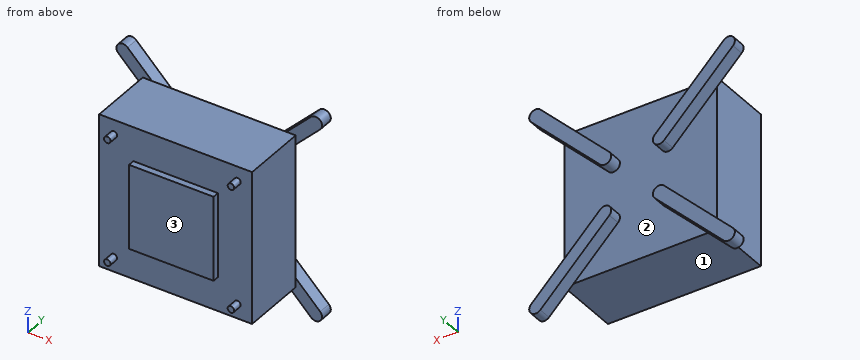
from build123d import *

# Parameters (mm, degrees)
ESQUISSE1_W        = 47
ESQUISSE1_H        = 47
BOSS_EXTRU_1_DEPTH = 20
ESQUISSE2_R        = 1
BOSS_EXTRU_2_DEPTH = 3
BOSS_EXTRU_3_DEPTH = 4
ESQUISSE4_W        = 26
ESQUISSE4_H        = 26
BOSS_EXTRU_4_DEPTH = 2


with BuildPart() as part:
    # Esquisse1 → Boss.-Extru.1 (new body)
    with BuildSketch(Plane(origin=(0, 0, 0), x_dir=(1, 0, 0), z_dir=(0, 1, 0))):
        Rectangle(ESQUISSE1_W, ESQUISSE1_H)
    extrude(amount=BOSS_EXTRU_1_DEPTH)

    # Esquisse2 → Boss.-Extru.2 (add)
    with BuildSketch(Plane.XZ):
        with Locations((19, -19)):
            Circle(ESQUISSE2_R)
        with Locations((-19, -19)):
            Circle(ESQUISSE2_R)
        with Locations((-19, 19)):
            Circle(ESQUISSE2_R)
        with Locations((19, 19)):
            Circle(ESQUISSE2_R)
    extrude(amount=BOSS_EXTRU_2_DEPTH)

    # Esquisse3 → Boss.-Extru.3 (add)
    with BuildSketch(Plane(origin=(0, 20, 0), x_dir=(1, 0, 0), z_dir=(0, 1, 0))):
        with BuildLine():
            Line((9.807611845, -6.97918472), (31.02081528, -28.192388155))
            ThreePointArc((31.02081528, -28.192388155), (31.02081528, -31.02081528), (28.192388155, -31.02081528))
            Line((28.192388155, -31.02081528), (6.97918472, -9.807611845))
            ThreePointArc((6.97918472, -9.807611845), (6.97918472, -6.97918472), (9.807611845, -6.97918472))
        make_face()
        with BuildLine():
            Line((9.807611845, 6.97918472), (31.02081528, 28.192388155))
            ThreePointArc((31.02081528, 28.192388155), (31.02081528, 31.02081528), (28.192388155, 31.02081528))
            Line((28.192388155, 31.02081528), (6.97918472, 9.807611845))
            ThreePointArc((6.97918472, 9.807611845), (6.97918472, 6.97918472), (9.807611845, 6.97918472))
        make_face()
        with BuildLine():
            Line((-9.807611845, -6.97918472), (-31.02081528, -28.192388155))
            ThreePointArc((-31.02081528, -28.192388155), (-31.02081528, -31.02081528), (-28.192388155, -31.02081528))
            Line((-28.192388155, -31.02081528), (-6.97918472, -9.807611845))
            ThreePointArc((-6.97918472, -9.807611845), (-6.97918472, -6.97918472), (-9.807611845, -6.97918472))
        make_face()
        with BuildLine():
            Line((-9.807611845, 6.97918472), (-31.02081528, 28.192388155))
            ThreePointArc((-31.02081528, 28.192388155), (-31.02081528, 31.02081528), (-28.192388155, 31.02081528))
            Line((-28.192388155, 31.02081528), (-6.97918472, 9.807611845))
            ThreePointArc((-6.97918472, 9.807611845), (-6.97918472, 6.97918472), (-9.807611845, 6.97918472))
        make_face()
    extrude(amount=BOSS_EXTRU_3_DEPTH)

    # Esquisse4 → Boss.-Extru.4 (add)
    with BuildSketch(Plane.XZ):
        Rectangle(ESQUISSE4_W, ESQUISSE4_H)
    extrude(amount=BOSS_EXTRU_4_DEPTH)


solid = part.part
Here's how the part is built. I have some questions about the finished solid (model axes, mm). Face numbers are marked on the shaded views. Round coordinates to 2 decimals unless told otherwise and drop trailing zeros. Order: outer loops, then holes, each group sorted by start corner. A loop starts at its lowest first (then second) coordinate and runs counter-clockwise, first axis right, second up. Notation, with made-up numbers: (-26.5, 72) -> (-8.5, 72) arc R30 cw to (-8.5, 97) -> close; hole circle Ø11 at (81, 28.5). An arc over 180 degrees is marked (long way). Return JSON: item names as keys, results as strings.
Q1. If we section it at C-C on z = -19: List the corners of the cut face in (x, y) for me, plus the area to 3 significant figures.
Filled sheet:
{"outline": "(-23.5, 0) -> (-20, 0) -> (-20, -3) -> (-18, -3) -> (-18, 0) -> (18, 0) -> (18, -3) -> (20, -3) -> (20, 0) -> (23.5, 0) -> (23.5, 20) -> (21.83, 20) -> (21.83, 24) -> (16.17, 24) -> (16.17, 20) -> (-16.17, 20) -> (-16.17, 24) -> (-21.83, 24) -> (-21.83, 20) -> (-23.5, 20) -> close", "area": "997 mm^2"}
Q2. If we section it at B-B on x = -2: List the corners of the cut face in (y, z) for me.
Filled sheet:
{"outline": "(-2, -13) -> (0, -13) -> (0, -23.5) -> (20, -23.5) -> (20, 23.5) -> (0, 23.5) -> (0, 13) -> (-2, 13) -> close"}
Q3. If we section it at D-D on y = 15: List the corners of the cut face in (x, z) for me.
Filled sheet:
{"outline": "(-23.5, -23.5) -> (23.5, -23.5) -> (23.5, 23.5) -> (-23.5, 23.5) -> close"}
Q4. I need wall thicknesses on line 1 along Z through (x, y) = (-21.5, 12.5); line 2 along Y through (x, z) = (-7, -2). Which ranges of each line are inside material? Lowest first, please. Write a range as from..to.
Filled sheet:
{"line 1": "z = -23.5..23.5", "line 2": "y = -2..20"}
Q5. If we section it at A-A on x = 27: List the corners of the cut face in (y, z) for me.
Filled sheet:
{"outline": "(20, -29.83) -> (24, -29.83) -> (24, -24.17) -> (20, -24.17) -> close; (20, 24.17) -> (24, 24.17) -> (24, 29.83) -> (20, 29.83) -> close"}
Q6. If we mould it in two halves opening along Z, with no side actions, what happens to the marked faces 1, 2 and 3? For each: released by +Z, released by -Z, zero draft, split by the parting line, or undercut.
Filled sheet:
{"face 1": "released by -Z", "face 2": "undercut", "face 3": "zero draft"}
Q7. For pin 1 Ø13 at (x, z) = (-3.5, 5) entering from -Y; pin 2 Ø6 at (x, y) = (-25, 7) entering from -Z; pin 3 Ø8 at (y, z) = (3.5, -5) entering from +X; pin 4 Ø12 at (x, z) = (-7, 17) entering from +Y, each with a flat end and sliding along its axis, tell me the tip position at first contact or that it passes through.
Filled sheet:
{"pin 1": "stops at y = -2", "pin 2": "stops at z = -23.5", "pin 3": "stops at x = 23.5", "pin 4": "stops at y = 24"}
